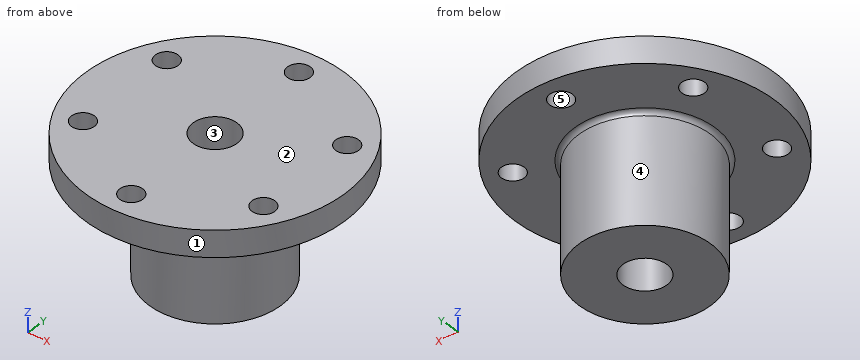
```python
from build123d import *

# Parameters (mm, degrees)
SKETCH1_R           = 29.5
SKETCH1_R_2         = 2.6
BOSS_EXTRUDE1_DEPTH = 6
SKETCH2_W           = 25
SKETCH2_H           = 15
FILLET1_R           = 1
SKETCH3_R           = 5
CUT_EXTRUDE1_DEPTH  = 31


with BuildPart() as part:
    # Sketch1 → Boss-Extrude1 (new body)
    with BuildSketch(Plane.XY):
        Circle(SKETCH1_R)
        with Locations((0, 23.75)):
            Circle(SKETCH1_R_2, mode=Mode.SUBTRACT)
        with Locations((20.56810334, 11.875)):
            Circle(SKETCH1_R_2, mode=Mode.SUBTRACT)
        with Locations((20.56810334, -11.875)):
            Circle(SKETCH1_R_2, mode=Mode.SUBTRACT)
        with Locations((0, -23.75)):
            Circle(SKETCH1_R_2, mode=Mode.SUBTRACT)
        with Locations((-20.56810334, -11.875)):
            Circle(SKETCH1_R_2, mode=Mode.SUBTRACT)
        with Locations((-20.56810334, 11.875)):
            Circle(SKETCH1_R_2, mode=Mode.SUBTRACT)
    extrude(amount=BOSS_EXTRUDE1_DEPTH)

    # Sketch2 → Revolve1 (revolve)
    with BuildSketch(Plane(origin=(0, 0, 0), x_dir=(0, 0, -1), z_dir=(1, 0, 0)), mode=Mode.PRIVATE) as revolve1_sk:
        with Locations((12.5, 7.5)):
            Rectangle(SKETCH2_W, SKETCH2_H)
    revolve(revolve1_sk.sketch.rotate(Axis((0, 0, 0), (0, 0, -1)), 90), axis=Axis((0, 0, 0), (0, 0, -1)))

    # Fillet1
    fillet1_edges = [part.edges().sort_by_distance(p)[0] for p in [
        (-15, 0, 0),
    ]]
    fillet(fillet1_edges, radius=FILLET1_R)

    # Sketch3 → Cut-Extrude1 (cut)
    with BuildSketch(Plane(origin=(0, 0, -25), x_dir=(-1, 0, 0), z_dir=(0, 0, -1))):
        Circle(SKETCH3_R)
    extrude(amount=-CUT_EXTRUDE1_DEPTH, mode=Mode.SUBTRACT)


solid = part.part
```
The model under review builds one solid part; all positions refer to its coordinate system, in mm. Face numbers are marked on the shaded views. A direction names the side the tool comes from. Round coordinates to 2 decimals unless told otherwise and drop trailing zeros. Write each loop counter-clockwise with the first axis right and the second up, starting at its lowest first coordinate (ties: lowest second). Pieces come first, ordered by that corner, then holes. Notation, with made-up numbers: (71.5, -8) - (117.5, -8) arc R32 ccw to (117.5, 29) - close; hole circle Ø7 at (-32.5, 0). An arc over 180 degrees is marked (long way). Answer as CSV lines item,"result". Start each with the question number.
(1) We need section D-D on z = -10.5. State the section outline as (x, y) points, plus the area to 3 significant figures.
(2) Draft analysis for pull direction Y (two halves, no side actions). For the marked faces 1, 2 and 3, state which applies: pulls with the +Y half, pulls with the -Y half, needs draft (parallel to the pull), parting line crosses it, or undercut.
(3) For the marked faces 4 and 5, list the 3-axis set-ups (+Z, -Z, +X, -X, +Y, -Y) from which the entire face can be reached by the end or side of a thin tool; tool diameter is ignored.
(4) We need section B-B on y = 0. State the section outline as (x, z) points.
(5) To check wall thickness, follow line 1 (Y direction, x = 19, z = 5.5); line 2 (Z direction, x = 18, y = 1); line 3 (X direction, y = 14, z = 4). State the ranges of each line that lie inside material, in increasing order.
(6) We need section C-C on x = -21.5. State the section outline as (y, z) points, plus the area to 3 significant figures.
(7) We need section A-A on x = 0. State the section outline as (y, z) points, plus the area to 3 significant figures.
(8) For pin 1 Ø10 at (y, z) = (-12.5, -10) entering from -X; pin 2 Ø12 at (y, z) = (-7, -7) entering from -X; pin 3 Ø6 at (x, y) = (20.57, 11.88) entering from -Z; pin 4 Ø9 at (x, y) = (0, 0) entering from +Z, all flat-tipped, find the tip position at first contact; note any pin that passes through.
Worked answers:
1,outline,"circle Ø30 at (0, 0); hole circle Ø10 at (0, 0)"
1,area,"628 mm²"
2,face 1,"parting line crosses it"
2,face 2,"needs draft"
2,face 3,"undercut"
3,face 4,"-Z"
3,face 5,"+Z, -Z"
4,outline,"(-29.5, 0) - (-16, 0) arc R1 cw to (-15, -1) - (-15, -25) - (-5, -25) - (-5, 6) - (-29.5, 6) - close; (5, -25) - (15, -25) - (15, -1) arc R1 cw to (16, 0) - (29.5, 0) - (29.5, 6) - (5, 6) - close"
5,line 1,"-22.57 to -13.95, -9.8 to 9.8, 13.95 to 22.57"
5,line 2,"0 to 6"
5,line 3,"-25.97 to -22.07, -19.07 to 19.07, 22.07 to 25.97"
6,outline,"(-20.2, 0) - (-14.3, 0) - (-14.3, 6) - (-20.2, 6) - close; (-9.45, 0) - (9.45, 0) - (9.45, 6) - (-9.45, 6) - close; (14.3, 0) - (20.2, 0) - (20.2, 6) - (14.3, 6) - close"
6,area,"184 mm²"
7,outline,"(-29.5, 0) - (-26.35, 0) - (-26.35, 6) - (-29.5, 6) - close; (-21.15, 0) - (-16, 0) arc R1 cw to (-15, -1) - (-15, -25) - (-5, -25) - (-5, 6) - (-21.15, 6) - close; (5, -25) - (15, -25) - (15, -1) arc R1 cw to (16, 0) - (21.15, 0) - (21.15, 6) - (5, 6) - close; (26.35, 0) - (29.5, 0) - (29.5, 6) - (26.35, 6) - close"
7,area,"732 mm²"
8,pin 1,"x = -12.99"
8,pin 2,"x = -14.97"
8,pin 3,"z = 0"
8,pin 4,"through"
